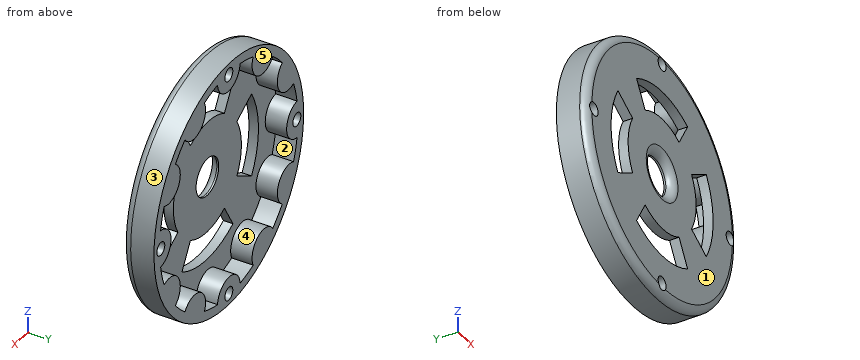
```python
from build123d import *

# Parameters (mm, degrees)
SKETCH1_R           = 41.91
BOSS_EXTRUDE3_DEPTH = 7.1501
BOSS_EXTRUDE4_START = -3.175
SKETCH1_8_R         = 41.91
BOSS_EXTRUDE4_DEPTH = 3.175
SKETCH3_R           = 6.35
CUT_EXTRUDE1_DEPTH  = 10.3251
CIRPATTERN1_COUNT   = 12
FILLET1_R           = 2.54
CUT_EXTRUDE2_REACH  = 62.162
SKETCH4_R           = 2.2225
CIRPATTERN2_COUNT   = 4
SCALE1_SCALE        = 2
CUT_EXTRUDE3_START  = -6.350001
CUT_EXTRUDE3_DEPTH  = 20.6502
CIRPATTERN3_COUNT   = 4
SCALE2_SCALE        = 0.5


with BuildPart() as part:
    # Sketch1 → Boss-Extrude3 (new body)
    with BuildSketch(Plane(origin=(0, 0, 0), x_dir=(1, 0, 0), z_dir=(0, 1, 0))):
        with Locations(Location((0, 0, 0), (0, 0, 270))):
            Circle(SKETCH1_R)
        with BuildLine():
            ThreePointArc((6.328632418, 38.214508197), (0, -38.735), (-6.328632418, 38.214508197))
            ThreePointArc((-6.328632418, 38.214508197), (0, 32.385), (6.328632418, 38.214508197))
        make_face(mode=Mode.SUBTRACT)
    boss_extrude3 = extrude(amount=BOSS_EXTRUDE3_DEPTH)

    # Sketch1<8> → Boss-Extrude4 (add)
    with BuildSketch(Plane(origin=(0, 0, 0), x_dir=(1, 0, 0), z_dir=(0, 1, 0)).offset(BOSS_EXTRUDE4_START)):
        with Locations(Location((0, 0, 0), (0, 0, 270))):
            Circle(SKETCH1_8_R)
    extrude(amount=BOSS_EXTRUDE4_DEPTH)

    # Sketch3 → Cut-Extrude1 (cut)
    with BuildSketch(Plane.XZ.offset(-7.1501)):
        with Locations(Location((0, 0, 0), (0, 0, 90))):
            Circle(SKETCH3_R)
    extrude(amount=CUT_EXTRUDE1_DEPTH, mode=Mode.SUBTRACT)

    # CirPattern1: Boss-Extrude3 ×12 about axis
    cirpattern1_axis = Axis((0, 0, 0), (0, 1, 0))
    for i in range(1, CIRPATTERN1_COUNT):
        add(boss_extrude3.rotate(cirpattern1_axis, i * 360 / CIRPATTERN1_COUNT))

    # Fillet1
    fillet1_edges = [part.edges().sort_by_distance(p)[0] for p in [
        (0, -3.175, -41.91),
        (0, -3.175, -6.35),
    ]]
    fillet(fillet1_edges, radius=FILLET1_R)

    # Cut-Extrude2: up to this face of the body (flat: up to its plane)
    cut_extrude2_end = Plane(part.part.faces().sort_by_distance((0, -3.175, -38.256448241))[0])
    # Sketch4 → Cut-Extrude2 (cut, up to the picked face)
    with BuildSketch(Plane(origin=(0, 7.1501, 0), x_dir=(1, 0, 0), z_dir=(0, 1, 0)), mode=Mode.PRIVATE) as cut_extrude2_sk1:
        with Locations(Location((0, 38.1, 0), (0, 0, 270))):
            Circle(SKETCH4_R)
    cut_extrude2_tool1 = split(extrude(cut_extrude2_sk1.sketch, amount=-CUT_EXTRUDE2_REACH, mode=Mode.PRIVATE), bisect_by=cut_extrude2_end, keep=Keep.BOTH, mode=Mode.PRIVATE)
    cut_extrude2 = cut_extrude2_tool1.solids().sort_by(Axis((0, 7.1501, -38.1), (0, -1, 0)))[0]
    add(cut_extrude2, mode=Mode.SUBTRACT)

    # CirPattern2: Cut-Extrude2 ×4 about axis
    cirpattern2_axis = Axis((0, 0, 0), (0, 1, 0))
    for i in range(1, CIRPATTERN2_COUNT):
        add(cut_extrude2.rotate(cirpattern2_axis, i * 360 / CIRPATTERN2_COUNT), mode=Mode.SUBTRACT)


with BuildPart() as part_1:
    # Scale1: scaled about (-1.3e-08, 0.44206654, 1e-09)
    add(part.part.scale(SCALE1_SCALE).moved(Location((1.3e-08, -0.44206654, -1e-09))))

    # Sketch5 → Cut-Extrude3 (cut)
    with BuildSketch(Plane(origin=(0, -0.442065876, 0), x_dir=(1, 0, 0), z_dir=(0, 1, 0)).offset(CUT_EXTRUDE3_START)):
        with BuildLine():
            Line((-19.05, 32.995567884), (-28.575, 49.493351826))
            ThreePointArc((-28.575, 49.493351826), (0, 57.15), (28.575, 49.493351826))
            Line((28.575, 49.493351826), (19.05, 32.995567884))
            ThreePointArc((19.05, 32.995567884), (0, 38.1), (-19.05, 32.995567884))
        make_face()
    cut_extrude3 = extrude(amount=CUT_EXTRUDE3_DEPTH, mode=Mode.SUBTRACT)

    # CirPattern3: Cut-Extrude3 ×4 about axis
    cirpattern3_axis = Axis((0, -6.792065876, 0), (0, 1, 0))
    for i in range(1, CIRPATTERN3_COUNT):
        add(cut_extrude3.rotate(cirpattern3_axis, i * 360 / CIRPATTERN3_COUNT), mode=Mode.SUBTRACT)


with BuildPart() as part_2:
    # Scale2: scaled about (-1.4e-08, 0.951448261, 2e-09)
    add(part_1.part.scale(SCALE2_SCALE).moved(Location((-7e-09, 0.475724131, 1e-09))))


solid = part_2.part
```
Design review of the part built by this model. Coordinates are the model's own, in mm. Face numbers are marked on the shaded views. A direction names the side the tool comes from. Round coordinates to 2 decimals unless told otherwise and drop trailing zeros. Put each result on its own line as item: value.
Q1. Insertion check: pin 1 Ø4 at (x, z) = (-38.1, 0) entering from +Y; pin 2 Ø4 at (y, z) = (-1.5, -31.5) entering from +X; pin 3 Ø4 at (y, z) = (3, 16) entering from +X; pin 4 Ø1.5 at (x, y) = (12.5, 4) entering from -Z. Each pin has a flat end and moves straight along its axis. Give the tip position at first contact, or say it passes through.
Reported:
pin 1: through
pin 2: x = 29.6
pin 3: x = 39.5
pin 4: z = -40.23
Q2. Consider section A-A (y = 2.5). State how many separate pieces and enclosed holes the cut face has, and give its area (3 significant figures).
Reported:
separate pieces: 1
enclosed holes: 5
area: 1,480 mm²
Q3. Draft analysis for pull direction Z (two halves, no side actions). For the marked faces 3, 4 and 5, state which applies: released by +Z, released by -Z, zero draft, split by the parting line, or undercut.
Reported:
face 3: split by the parting line
face 4: undercut
face 5: zero draft
Q4. Machinability: for the marked faces 1 and 2, which of the approach directions +Z, -Z, +X, -X, +Y, -Y give a long, thin tool a straight path to every point of the face, cutting with its end or side? Answer none if there is none.
Reported:
face 1: +Z, -Z, +X, -X, -Y
face 2: +Y
Q5. To check wall thickness, follow line 1 (Z direction, x = -1, y = -0.25); line 2 (Y direction, x = 31, z = -9.5); line 3 (X direction, y = 6.5, z = -35). State the ranges of each line that lie inside material, in increasing order.
Reported:
line 1: -41.9 to -40.08, -36.12 to -28.56, -19.02 to -6.27, 6.27 to 19.02, 28.56 to 36.12, 40.08 to 41.9
line 2: -2.92 to 0.25
line 3: -23.05 to -13.19, -5.14 to 5.14, 13.19 to 23.05
